Source: CAD feature listing. Evaluate the final solid. Frame: model axes, mm. Face numbers are marked on the shaded views. Give positions to 0.01 mm unless a question says otherwise; leave off trailing zeros. Loops run counter-clockwise (first coordinate to the right, second up) from the corner with the lowest first, then second, coordinate; pieces in that order, holes last. Notation, with made-up numbers: M -5.5,82.25 L 13.5,82.25 A30 cw 13.5,112.25 Z; hole C 30,49.5 d5. An arc over 180 degrees is marked long. Put each result on its own line as item: value. Start each with the question number.
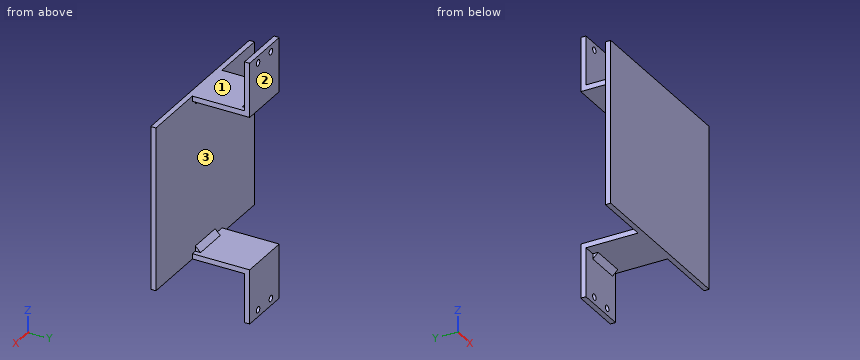
```python
from build123d import *

# Parameters (mm, degrees)
SKETCH1_W           = 100
SKETCH1_H           = 94
BOSS_EXTRUDE1_DEPTH = 3
SKETCH2_W           = 30
SKETCH2_H           = 3
BOSS_EXTRUDE2_DEPTH = 33
BOSS_EXTRUDE3_DEPTH = 10
SKETCH4_W           = 30
SKETCH4_H           = 28.25
SKETCH4_R           = 1.75
BOSS_EXTRUDE4_DEPTH = 3


with BuildPart() as part:
    # Sketch1 → Boss-Extrude1 (new body)
    with BuildSketch(Plane(origin=(0, 0, 0), x_dir=(1, 0, 0), z_dir=(0, 1, 0))):
        Rectangle(SKETCH1_W, SKETCH1_H)
    extrude(amount=-BOSS_EXTRUDE1_DEPTH)

    # Sketch2 → Boss-Extrude2 (add)
    with BuildSketch(Plane(origin=(0, 0, 0), x_dir=(1, 0, 0), z_dir=(0, 1, 0))):
        with Locations((-2, 45.5)):
            Rectangle(SKETCH2_W, SKETCH2_H)
        with Locations((-2, -45.5)):
            Rectangle(SKETCH2_W, SKETCH2_H)
    extrude(amount=BOSS_EXTRUDE2_DEPTH)

    # Sketch3 → Boss-Extrude3 (add, symmetric)
    with BuildSketch(Plane(origin=(0, 0, 0), x_dir=(0, 0, -1), z_dir=(1, 0, 0))):
        Polygon((-44, 3), (-41, 0), (-44, 0), align=None)
        Polygon((44, 3), (41, 0), (44, 0), align=None)
        Polygon((-47, 30), (-50, 30), (-47, 27), align=None)
        Polygon((47, 30), (47, 27), (50, 30), align=None)
    extrude(amount=BOSS_EXTRUDE3_DEPTH, both=True)

    # Sketch4 → Boss-Extrude4 (add)
    # profile 1 of 2: a face of its own
    with BuildSketch(Plane(origin=(0, 33, 0), x_dir=(1, 0, 0), z_dir=(0, 1, 0))):
        with Locations((-2, 61.125)):
            Rectangle(SKETCH4_W, SKETCH4_H)
        with Locations(Location((-8.5, 71.25, 0), (0, 0, 270))):
            Circle(SKETCH4_R, mode=Mode.SUBTRACT)
        with Locations(Location((4.5, 71.25, 0), (0, 0, 270))):
            Circle(SKETCH4_R, mode=Mode.SUBTRACT)
    # profile 2 of 2: a face of its own
    with BuildSketch(Plane(origin=(0, 33, 0), x_dir=(1, 0, 0), z_dir=(0, 1, 0))):
        with Locations((-2, -61.125)):
            Rectangle(SKETCH4_W, SKETCH4_H)
        with Locations(Location((-8.5, -71.25, 0), (0, 0, 270))):
            Circle(SKETCH4_R, mode=Mode.SUBTRACT)
        with Locations(Location((4.5, -71.25, 0), (0, 0, 270))):
            Circle(SKETCH4_R, mode=Mode.SUBTRACT)
    extrude(amount=-BOSS_EXTRUDE4_DEPTH)


solid = part.part
```
1. Section D-D, the plane z = 17. Output: boundary loops of the cut face in (x, y).
2. Pull-direction query (Z, two-part tool) for the marked faces 1, 2 and 3; classes: released by +Z, released by -Z, zero draft, split by the parting line, or undercut.
3. Ray query, line 1 (X direction, y = 31, z = 71.25); line 2 (Z direction, x = -7, y = 24); line 3 (Z direction, x = 4, y = 31). Return the intervals inside material, ascending.
4. Section B-B, the plane y = 5. Output: boundary loops of the cut face in (x, z), plus the area to 3 significant figures.
5. Contact query for flat-ended pins moving along their axis: pin 1 (12 mm diameter, centred on y = 13.5, z = 50.5, fed in from +X); pin 2 (16.5 mm diameter, centred on x = -11.5, y = 5.5, fed in from +Z); pin 3 (0.9 mm diameter, centred on y = 1, z = -42, fed in from -X). Output: stop coordinate, or through.
6. Section C-C, the plane z = 71.25. Output: boundary loops of the cut face in (x, y).
7. Section A-A, the plane x = 4.5. Output: boundary loops of the cut face in (y, z).
Results found:
1. outline: M -50,-3 L 50,-3 L 50,0 L -50,0 Z
2. face 1: released by +Z
2. face 2: zero draft
2. face 3: undercut
3. line 1: -17 to -10.25, -6.75 to 2.75, 6.25 to 13
3. line 2: -47 to -44, 44 to 47
3. line 3: -75.25 to -72.93, -69.57 to -44, 44 to 69.57, 72.93 to 75.25
4. outline: M -17,-47 L 13,-47 L 13,-44 L -17,-44 Z; M -17,44 L 13,44 L 13,47 L -17,47 Z
4. area: 180 mm²
5. pin 1: x = 13
5. pin 2: z = 47
5. pin 3: x = -10
6. outline: M -17,30 L -10.25,30 L -10.25,33 L -17,33 Z; M -6.75,30 L 2.75,30 L 2.75,33 L -6.75,33 Z; M 6.25,30 L 13,30 L 13,33 L 6.25,33 Z
7. outline: M -3,-47 L 27,-47 L 30,-50 L 30,-69.5 L 33,-69.5 L 33,-44 L 3,-44 L 0,-41 L 0,41 L 3,44 L 33,44 L 33,69.5 L 30,69.5 L 30,50 L 27,47 L -3,47 Z; M 30,-75.25 L 33,-75.25 L 33,-73 L 30,-73 Z; M 30,73 L 33,73 L 33,75.25 L 30,75.25 Z
